Could you check a few things on this model? Use its own coordinates, in mm. Face numbers are marked on the shaded views. A direction names the side the tool comes from. Round coordinates to 2 decimals unless told otherwise and drop trailing zeros. Loops run counter-clockwise (first coordinate to the right, second up) from the corner with the lowest first, then second, coordinate; pieces in that order, holes last. Notation, with made-up numbers: (55, 71.5) -> (61, 71.5) arc R27 cw to (61, 90.5) -> close; hole circle Ø2 at (-4.5, 73). An arc over 180 degrees is marked (long way). Write each question's results on one line, items separated by ' | '. Start each with the question number.
1) Imagine slicing it at A-A, the plane z = 18. Give the number of separate pieces and of enclosed holes in the cut face, plus the area to 3 significant figures.
2) For P1, Ø8, axis at y = 473, z = 13, coming from the -X side; P2, Ø3, axis at x = 286.5, z = 35.5, coming from the -Y side; P3, Ø8, axis at x = 325.5, z = 21, coming from the -Y side, each with a flat end and sliding along its axis, tell me the tip position at first contact or that it passes through.
3) Which directions (+Z, -Z, +X, -X, +Y, -Y) give clear straight access to the entire face, cutting with the end or side of a thin tool? Please do the marked faces 1, 2 and 3.
4) Imagine slicing it at B-B, the plane y = 408. List the corners of the cut face in (x, z) for me, plus the area to 3 significant figures.
5) If I drill on probe 1 along Y at (x, z) = (274.5, 31.5); probe 2 along Y at (x, z) = (272, 36.5); probe 3 along X at (y, z) = (227.5, 26.5), over which ranges is the centre line in solid material (lowest first)?
6) We'd pull the mould along X, two halves only. Please class the marked faces 4, 5 and 6: pulls with the +X half, pulls with the -X half, needs draft (parallel to the pull), parting line crosses it, or undercut.
7) Imagine slicing it at C-C, the plane y = 482. List the corners of the cut face in (x, z) for me, plus the area to 3 significant figures.
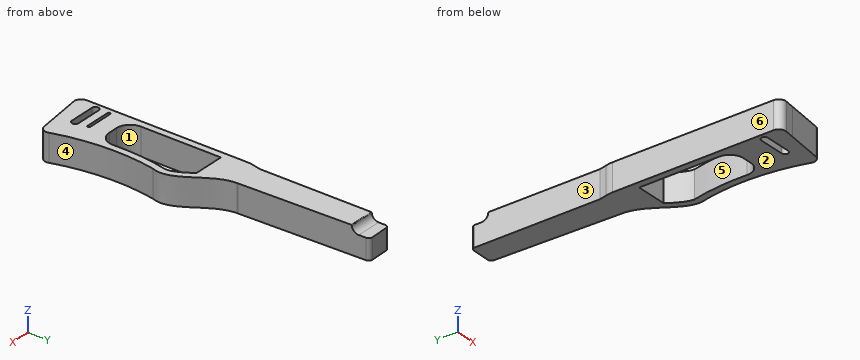
from build123d import *

# Parameters (mm, degrees)
BOSS_EXTRUDE3_DEPTH = 40
CUT_EXTRUDE1_START  = -10
CUT_EXTRUDE1_DEPTH  = 10
FILLET3_R           = 10
FILLET4_R           = 1
CUT_EXTRUDE3_DEPTH  = 634.823473561


with BuildPart() as part:
    # Sketch1 → Boss-Extrude3 (new body)
    with BuildSketch(Plane.XY):
        with BuildLine():
            Line((287.157860281, 534.451448831), (260.19721277, 533.779001198))
            ThreePointArc((260.19721277, 533.779001198), (256.742542962, 532.271733759), (255.321883101, 528.780555709))
            Line((255.321883101, 528.780555709), (255.321883101, 346.027702032))
            Line((255.321883101, 346.027702032), (255.321883101, 298.309919691))
            Line((255.321883101, 298.309919691), (298.321883101, 298.309919691))
            Line((298.321883101, 298.309919691), (297.107965759, 344.783089771))
            add(Edge.make_bspline(
                [(297.107965759, 344.783089771), (297.092597, 345.195665623), (297.081725868, 345.610516215), (297.075455466, 346.027702032)],
                knots=[0.989098045, 0.989098045, 0.989098045, 0.989098045, 1, 1, 1, 1], degree=3))
            Line((297.075455466, 346.027702032), (292.280825741, 529.583562912))
            ThreePointArc((292.280825741, 529.583562912), (290.726675353, 533.077622908), (287.157860281, 534.451448831))
        make_face()
        with BuildLine():
            Line((255.321883101, 298.309919691), (255.321883101, 346.027702032))
            add(Edge.make_bspline(
                [(255.321883101, 346.027702032), (254.757957002, 342.410351737), (253.98676421, 338.857518857), (253.008304725, 335.36920339)],
                knots=[0, 0, 0, 0, 0.135221531, 0.135221531, 0.135221531, 0.135221531], degree=3))
            ThreePointArc((253.008304725, 335.36920339), (251.895242603, 330.018633631), (251.521898803, 324.566283821))
            Line((251.521898803, 324.566283821), (251.521898803, 112.494253422))
            Line((251.521898803, 112.494253422), (251.521898803, 107.975148622))
            Line((251.521898803, 107.975148622), (251.521898803, 107.687415528))
            Line((251.521898803, 107.687415528), (251.521898803, 107.377085198))
            Line((251.521898803, 107.377085198), (251.521898803, 89.434656666))
            ThreePointArc((251.521898803, 89.434656666), (254.924316425, 81.919877444), (262.816280156, 79.518781671))
            Line((262.816280156, 79.518781671), (276.783936318, 81.342067431))
            Line((276.783936318, 81.342067431), (329.661316312, 88.244483474))
            ThreePointArc((329.661316312, 88.244483474), (336.875168963, 92.905840971), (337.812674038, 101.443346932))
            ThreePointArc((337.812674038, 101.443346932), (325.065095163, 174.067394927), (330.156614349, 247.625736037))
            add(Edge.make_bspline(
                [(330.156614349, 247.625736037), (336.006706917, 262.277420591), (320.933871266, 296.427871643), (297.92215095, 322.926208236), (297.107965759, 344.783089771)],
                knots=[0, 0, 0, 0, 0.411549101, 0.989098045, 0.989098045, 0.989098045, 0.989098045], degree=3))
            Line((297.107965759, 344.783089771), (298.321883101, 298.309919691))
            Line((298.321883101, 298.309919691), (255.321883101, 298.309919691))
        make_face()
    extrude(amount=BOSS_EXTRUDE3_DEPTH)

    # Sketch3 → Cut-Extrude1 (cut)
    with BuildSketch(Plane.XY.offset(40).offset(CUT_EXTRUDE1_START)):
        with BuildLine():
            Line((255.321883101, 508.869919691), (292.821883101, 508.869919691))
            Line((292.821883101, 508.869919691), (292.280825741, 529.583562912))
            ThreePointArc((292.280825741, 529.583562912), (290.726675353, 533.077622908), (287.157860281, 534.451448831))
            Line((287.157860281, 534.451448831), (260.19721277, 533.779001198))
            ThreePointArc((260.19721277, 533.779001198), (256.742542962, 532.271733759), (255.321883101, 528.780555709))
            Line((255.321883101, 528.780555709), (255.321883101, 508.869919691))
        make_face()
        with BuildLine():
            Line((260.321883101, 126.869919691), (297.821883101, 126.869919691))
            ThreePointArc((297.821883101, 126.869919691), (299.821883101, 128.869919691), (297.821883101, 130.869919691))
            Line((297.821883101, 130.869919691), (260.321883101, 130.869919691))
            ThreePointArc((260.321883101, 130.869919691), (258.321883101, 128.869919691), (260.321883101, 126.869919691))
        make_face()
    extrude(amount=CUT_EXTRUDE1_DEPTH, mode=Mode.SUBTRACT)

    # Fillet3
    fillet3_edges = [part.edges().sort_by_distance(p)[0] for p in [
        (274.071883101, 508.869919691, 30),
    ]]
    fillet(fillet3_edges, radius=FILLET3_R - 0.0001)  # a hair under: the kernel refuses the full size

    # Fillet4
    fillet4_edges = [part.edges().sort_by_distance(p)[0] for p in [
        (274.071883101, 508.869919691, 40),
    ]]
    fillet(fillet4_edges, radius=FILLET4_R)

    # Sketch7 → Cut-Extrude3 (cut, through all)
    with BuildSketch(Plane.XY):
        with BuildLine():
            Line((261.521898803, 105.235423074), (299.520758285, 105.235423074))
            ThreePointArc((299.520758285, 105.235423074), (304.415246799, 110.129911588), (299.520758285, 115.024400103))
            Line((299.520758285, 115.024400103), (261.521898803, 115.024400103))
            ThreePointArc((261.521898803, 115.024400103), (256.627410288, 110.129911588), (261.521898803, 105.235423074))
        make_face()
        with BuildLine():
            Line((307.783918876, 293.411121556), (261.521898803, 293.411121556))
            Line((261.521898803, 293.411121556), (261.521898803, 176.49325551))
            ThreePointArc((261.521898803, 176.49325551), (267.379763179, 162.351119886), (281.521898803, 156.49325551))
            Line((281.521898803, 156.49325551), (294.92087878, 156.49325551))
            ThreePointArc((294.92087878, 156.49325551), (309.345533596, 162.639399244), (314.90458823, 177.300322166))
            ThreePointArc((314.90458823, 177.300322166), (315.963249783, 218.705128996), (322.4563298, 259.611347408))
            add(Edge.make_bspline(
                [(322.4563298, 259.611347408), (322.456016347, 259.894497294), (322.421435552, 261.716157514), (321.977489562, 265.178835066), (320.516125801, 270.243060555), (318.282615138, 275.554318374), (315.425430629, 281.021812849), (312.162343995, 286.528772314), (309.555661166, 290.650913462), (308.084642597, 292.943229146), (307.783918876, 293.411121556)],
                knots=[0.113442682, 0.113442682, 0.113442682, 0.113442682, 0.125, 0.1875, 0.25, 0.3125, 0.375, 0.4375, 0.498593555, 0.514218555, 0.514218555, 0.514218555, 0.514218555], degree=3))
        make_face()
    extrude(amount=CUT_EXTRUDE3_DEPTH, mode=Mode.SUBTRACT)


solid = part.part
Checked values:
1) separate pieces: 1 | enclosed holes: 2 | area: 18,600 mm^2
2) P1: x = 255.32 | P2: y = 82.41 | P3: y = 87.18
3) face 1: +Z, -Z | face 2: -Z, +X, -X, +Y, -Y | face 3: +Z, -Z, -X, +Y
4) outline: (255.32, 0) -> (295.46, 0) -> (295.46, 40) -> (255.32, 40) -> close | area: 1,610 mm^2
5) probe 1: 81.04 to 105.24, 115.02 to 126.87, 130.87 to 157.77, 293.41 to 513.6 | probe 2: 80.72 to 105.24, 115.02 to 126.87, 130.87 to 158.91, 293.41 to 509.5 | probe 3: 251.52 to 261.52, 316.9 to 326.97
6) face 4: pulls with the +X half | face 5: undercut | face 6: pulls with the -X half
7) outline: (255.32, 0) -> (293.52, 0) -> (293.52, 40) -> (255.32, 40) -> close | area: 1,530 mm^2
